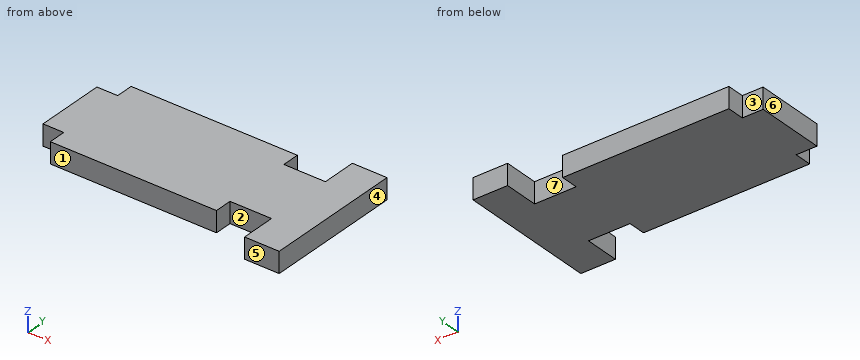
```python
from build123d import *

# Parameters (mm, degrees)
ESBO_O1_W                = 3
ESBO_O1_H                = 10
ESBO_O1_W_2              = 6
RESSALTO_EXTRUS_O1_DEPTH = 3


with BuildPart() as part:
    # Esboço1 → Ressalto-extrusão1 (new body)
    with BuildSketch(Plane.XY):
        Polygon((-12, -5), (-12, -7.5), (12, -7.5), (12, -5), (12, 5), (12, 7.5), (-12, 7.5), (-12, 5), align=None)
        with Locations((-13.5, 0)):
            Rectangle(ESBO_O1_W, ESBO_O1_H)
        with Locations((15, 0)):
            Rectangle(ESBO_O1_W_2, ESBO_O1_H)
        Polygon((18, 5), (18, -5), (18, -10), (23, -10), (23, 10), (18, 10), align=None)
    extrude(amount=RESSALTO_EXTRUS_O1_DEPTH)


solid = part.part
```
Here's how the part is built. I have some questions about the finished solid (model axes, mm). Face numbers are marked on the shaded views. A direction names the side the tool comes from. Round coordinates to 2 decimals unless told otherwise and drop trailing zeros. Order: outer loops, then holes, each group sorted by start corner. A loop starts at its lowest first (then second) coordinate and runs counter-clockwise, first axis right, second up. Notation, with made-up numbers: M 42.25,-25.75 L 53.25,-25.75 A16 cw 53.25,-17.75 Z; hole C 87,56 d11. An arc over 180 degrees is marked long. Use CSV: the item, a comma, the result in double quotes.
1) On a 3-axis mill with a long thin cutter (end or side, diameter ignored), from which of +Z, -Z, +X, -X, +Y, -Y can I reach the whole of each face in a straight line? I mean the marked faces 1, 2 and 3. Say none if no direction works.
Taken from the geometry:
face 1,"+Z, -Z, -X, -Y"
face 2,"+Z, -Z, -Y"
face 3,"+Z, -Z, -X, +Y"
2) I want a section at B-B (z = 1.75). List the corners of the cut face in (x, y) for me, then the cut area to 3 significant figures.
Taken from the geometry:
outline,"M -15,-5 L -12,-5 L -12,-7.5 L 12,-7.5 L 12,-5 L 18,-5 L 18,-10 L 23,-10 L 23,10 L 18,10 L 18,5 L 12,5 L 12,7.5 L -12,7.5 L -12,5 L -15,5 Z"
area,"550 mm^2"
3) I want a section at A-A (y = 6). List the corners of the cut face in (x, z) for me.
Taken from the geometry:
outline,"M -12,0 L 12,0 L 12,3 L -12,3 Z; M 18,0 L 23,0 L 23,3 L 18,3 Z"
4) If we mould it in two halves opening along X, with no side actions, what happens to the marked faces 4, 5, 6 and 7? For each: pulls with the +X half, pulls with the -X half, needs draft (parallel to the pull), parting line crosses it, or undercut.
Taken from the geometry:
face 4,"pulls with the +X half"
face 5,"needs draft"
face 6,"pulls with the -X half"
face 7,"undercut"
5) I'm going to push flat-ended pins straight in: P1, Ø1, axis at y = -7.5, z = 1.5, coming from the -X side; P2, Ø0.9, axis at y = 8.5, z = 1.5, coming from the -X side; P3, Ø1.5, axis at x = 6.5, z = 2.5, coming from the -Y side. Where does each tip first touch, or does it pass through?
Taken from the geometry:
P1,"x = -12"
P2,"x = 18"
P3,"y = -7.5"
6) I want a section at D-D (x = 1.5). List the corners of the cut face in (y, z) for me, then the cut area to 3 significant figures.
Taken from the geometry:
outline,"M -7.5,0 L 7.5,0 L 7.5,3 L -7.5,3 Z"
area,"45.0 mm^2"
7) I need wall thicknesses on line 1 along X through (y, z) = (-6.5, 0.35); line 2 along Y through (x, z) = (-2.5, 2.2); line 3 along X through (y, z) = (8.75, 2.95). Which ranges of each line are inside material? Lowest first, please. Write a range as [from, to].
Taken from the geometry:
line 1,"[-12, 12], [18, 23]"
line 2,"[-7.5, 7.5]"
line 3,"[18, 23]"
8) I want a section at C-C (x = 15). List the corners of the cut face in (y, z) for me.
Taken from the geometry:
outline,"M -5,0 L 5,0 L 5,3 L -5,3 Z"
